```python
from build123d import *

# Parameters (mm, degrees)
F0_W     = 96.186884
F0_H     = 94.729506
F1_DEPTH = 25
F2_W     = 11.076067
F2_H     = 8.452787
F3_DEPTH = 1
F4_W     = 96.186884
F4_H     = 94.729506
F5_DEPTH = 12.5
F6_R     = 1.955277
F7_DEPTH = 12.5


with BuildPart() as f1:
    # F0 (on Front) → F1 (new body)
    with BuildSketch(Plane.XZ):
        Rectangle(F0_W, F0_H)
    extrude(amount=-F1_DEPTH)

    # F2 (on face) → F3 (join)
    with BuildSketch(Plane(origin=(-48.093442, 0, 0), x_dir=(0, -1, 0), z_dir=(-1, 0, 0))):
        with Locations((-13.99082, 4.226393)):
            Rectangle(F2_W, F2_H)
    extrude(amount=F3_DEPTH)

    # F4 (on face) → F5 (join, symmetric)
    with BuildSketch(Plane(origin=(0, 25, 0), x_dir=(-1, 0, 0), z_dir=(0, 1, 0))):
        Rectangle(F4_W, F4_H)
    extrude(amount=F5_DEPTH, both=True)

    # F6 (on face) → F7 (cut, symmetric)
    with BuildSketch(Plane(origin=(-48.093442, 0, 0), x_dir=(0, -1, 0), z_dir=(-1, 0, 0))):
        with Locations((-13.99082, 4.809345)):
            Circle(F6_R)
    extrude(amount=F7_DEPTH, both=True, mode=Mode.SUBTRACT)


solid = f1.part
```
Part model, mm, in its own coordinate system. A direction names the side the tool comes from. Round coordinates to 2 decimals unless told otherwise and drop trailing zeros. Return JSON: item names as keys, results as strings. Group by question number.
Q1. Mould opens along Z. For faces 1 (the flat face through (-1, 18, 47.365)), 2 (the flat face through (-49.093, 14, 2)), 3 (the flat face through (-1, 18, -47.365)), 4 (the flat face through (-35.593, 14, 5)) say: pulls with the +Z half, pulls with the -Z half, needs draft (parallel to the pull), parting line crosses it, or undercut.
Q2. Probe L1, parallel to X at y = 17, z = -14. List the from-to ranges inside material, lowest first. Write a range as [from, to].
Q3. Which spindle directions (+Z, -Z, +X, -X, +Y, -Y) get a long thin tool onto all of the face, cutting with end or side? Do faces 5 (the cylindrical face through (-42.438, 12.185, 4.06)), 6 (the flat face through (-1, 0, 1)). Say none if no direction does.
Q4. Pin check, flat tip, straight feed: pin 1 (12 mm diameter, centred on y = 9, z = -12, fed in from -X). Stop position of the tip, or through.
Answer:
{
 "1": {"face 1": "pulls with the +Z half", "face 2": "needs draft", "face 3": "pulls with the -Z half", "face 4": "undercut"},
 "2": {"L1": "[-48.09, 48.09]"},
 "3": {"face 5": "-X", "face 6": "+Z, -Z, +X, -X, -Y"},
 "4": {"pin 1": "x = -48.09"}
}
